Build history of the part. All positions in model axes, mm. Face numbers are marked on the shaded views. Give positions to 0.01 mm unless a question says otherwise; leave off trailing zeros. Loops run counter-clockwise (first coordinate to the right, second up) from the corner with the lowest first, then second, coordinate; pieces in that order, holes last. Notation, with made-up numbers: (0.5, 83) -> (25.5, 83) arc R24 ccw to (25.5, 97) -> close; hole circle Ø3 at (4.5, -16.75). An arc over 180 degrees is marked (long way). Answer as a JSON object with one key per item and string values. Group by question number.
Q1. Wall check: probe 1 along Y at (x, z) = (-10, -26); probe 2 along Z at (x, y) = (-9, 17); probe 3 along X at (y, z) = (30.4, 0). Give the ranges that are in metal, low to high. Write a range as from..to.
Q2. Band-saw the part on A-A, the plane x = 0. Write the cut outline in (y, z), plus the area to 3 significant figures.
Q3. Band-saw the part on C-C, the plane y = 20. Write the cut outline in (x, z), plus the area to 3 significant figures.
Q4. Drop flat-ended pins along their axis: pin 1 (8 mm diameter, centred on y = 15, z = -12.5, fed in from +X); pin 2 (8 mm diameter, centred on y = 7.5, z = 10.5, fed in from +X); pin 3 (12 mm diameter, centred on x = -4.5, y = 8.5, fed in from -Z). Give the stop position or say it passes through.
Q5. Two-plate mould, pull along Z, no slides. Class the marked faces 1, 2, 3 and 4: pulls with the +Z half, pulls with the -Z half, needs draft (parallel to the pull), parting line crosses it, or undercut.
Q6. Band-saw the part on B-B, the plane y = 5.5. Write the cut outline in (x, z).
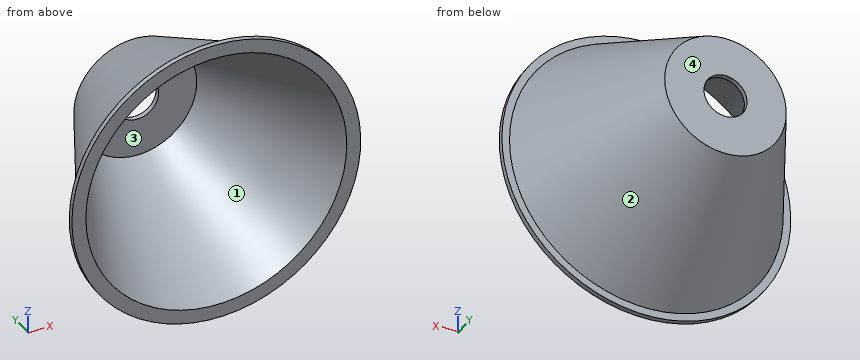
from build123d import *

# Parameters (mm, degrees)
SKETCH1_R           = 28.5
BOSS_EXTRUDE1_DEPTH = 1
SKETCH8_R           = 27
SKETCH3_R           = 12
SKETCH9_R           = 25.75
CUT_EXTRUDE1_DEPTH  = 30
CUT_EXTRUDE1_DRAFT  = -25
SKETCH10_R          = 4.25
CUT_EXTRUDE2_DEPTH  = 5


with BuildPart() as part:
    # Sketch1 → Boss-Extrude1 (new body)
    with BuildSketch(Plane(origin=(0, 0, 0), x_dir=(1, 0, 0), z_dir=(0, 1, 0))):
        with Locations(Location((0, 0, 0), (0, 0, 270))):
            Circle(SKETCH1_R)
    extrude(amount=BOSS_EXTRUDE1_DEPTH)

    # Sketch8 → Loft2 section 0
    with BuildSketch(Plane(origin=(0, 1, 0), x_dir=(1, 0, 0), z_dir=(0, 1, 0))):
        Circle(SKETCH8_R)
    # Sketch3 → Loft2 section 1
    with BuildSketch(Plane(origin=(0, 31, 0), x_dir=(1, 0, 0), z_dir=(0, 1, 0))):
        Circle(SKETCH3_R)
    loft()


with BuildPart() as cut_extrude1_tool:
    # Sketch9 → Cut-Extrude1 (with draft: the straight prism first)
    with BuildSketch(Plane.XZ):
        Circle(SKETCH9_R)
    extrude(amount=-CUT_EXTRUDE1_DEPTH)
    # Cut-Extrude1: the draft: its side faces are tilted about the plane it starts from
    cut_extrude1_sides = [cut_extrude1_tool.faces().sort_by_distance(p)[0] for p in [
        (-25.75, 15, 0),
    ]]
    draft(cut_extrude1_sides, Plane.XZ, CUT_EXTRUDE1_DRAFT)


with BuildPart() as part_1:
    add(part.part)

    # Cut-Extrude1: cut by cut_extrude1_tool
    add(cut_extrude1_tool.part, mode=Mode.SUBTRACT)

    # Sketch10 → Cut-Extrude2 (cut)
    with BuildSketch(Plane.XZ.offset(-30)):
        with Locations(Location((0, 0, 0), (0, 0, 270))):
            Circle(SKETCH10_R)
    extrude(amount=-CUT_EXTRUDE2_DEPTH, mode=Mode.SUBTRACT)


solid = part_1.part
Worked answers:
{
 "1": {"probe 1": "0..1", "probe 2": "-16.73..-15.38, 15.38..16.73", "probe 3": "-12.3..-4.25, 4.25..12.3"},
 "2": {"outline": "(0, -28.5) -> (1, -28.5) -> (1, -27) -> (31, -12) -> (31, -4.25) -> (30, -4.25) -> (30, -11.76) -> (0, -25.75) -> close; (0, 25.75) -> (30, 11.76) -> (30, 4.25) -> (31, 4.25) -> (31, 12) -> (1, 27) -> (1, 28.5) -> (0, 28.5) -> close", "area": "93.2 mm2"},
 "3": {"outline": "circle Ø35 at (0, 0); hole circle Ø32.85 at (0, 0)", "area": "115 mm2"},
 "4": {"pin 1": "x = 19.11", "pin 2": "x = 24.03", "pin 3": "z = -25.98"},
 "5": {"face 1": "undercut", "face 2": "parting line crosses it", "face 3": "undercut", "face 4": "needs draft"},
 "6": {"outline": "circle Ø49.5 at (0, 0); hole circle Ø46.37 at (0, 0)"}
}
